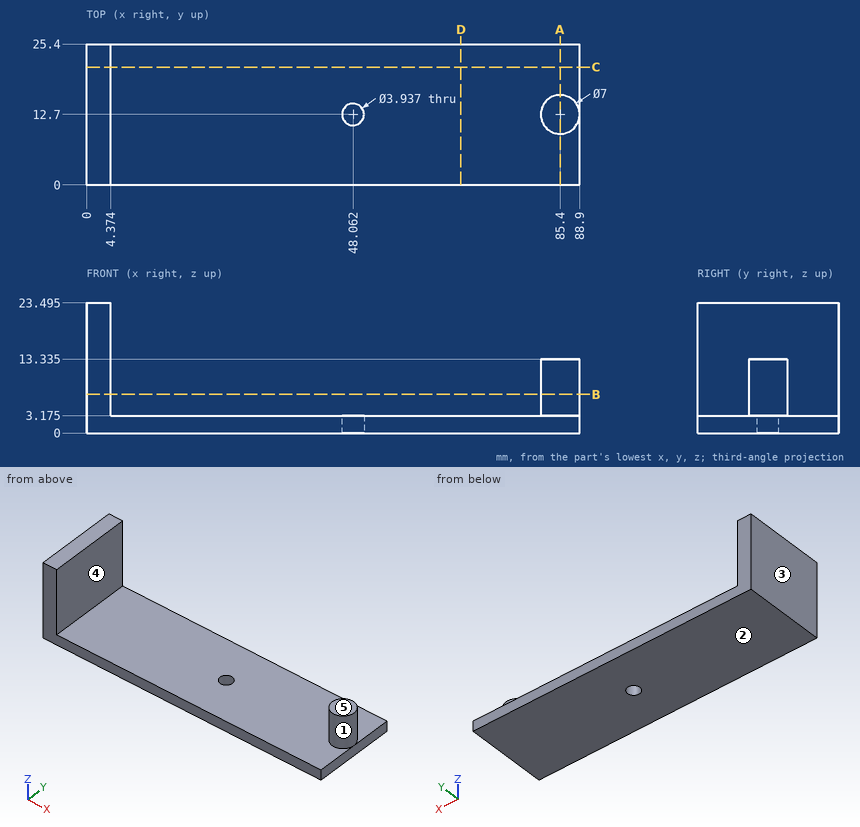
Answer from the drawing. Dimensions are ordinates in mm from the lowest x, y and z of the part. A direction names the side the tool comes from. Round coordinates to 2 decimals unless told otherwise and drop trailing zeros. Order: outer loops, then holes, each group sorted by start corner. A loop starts at its lowest first (then second) coordinate and runs counter-clockwise, first axis right, second up.
1) For the marked faces 4 and 5, determine the directions among +Z, -Z, +X, -X, +Y, -Y from which every point of the face is accessible in a straight line to the end or side of a thin tool.
2) The part is cut by section A-A on x = 85.4. Write down the section's boundary in (y, z) (3 decimals).
3) The part is cut by section C-C on y = 21.25. Write down the section's boundary in (x, z) (3 decimals).
4) The mould has two halves that part along X. Classify the marked faces 1, 2 and 3: released by +X, released by -X, zero draft, split by the parting line, or undercut.
5) Flat-ended cylindrical pins translate along their axes: pin 1 (7.5 mm diameter, centred on x = 86, y = 11.5, fed in from +Z) (3 decimals); pin 2 (2 mm diameter, centred on y = 20, z = 7.5, fed in from +X); pin 3 (7.5 mm diameter, centred on x = 48, y = 13.5, fed in from +Z) (3 decimals). Find the tip coordinate at first contact, or state that the pin passes through.
6) The part is cut by section B-B on z = 7. Write down the section's boundary in (x, y), plus the area to 3 significant figures.
7) The part is cut by section D-D on x = 67.5. Write down the section's boundary in (y, z) (3 decimals).
8) Straight lines are drawn through the part: L1, parallel to Z at x = 8.5, y = 14.5 (3 decimals); L2, parallel to X at y = 4.5, z = 7; L3, parallel to X at y = 13.5, z = 5.25. For each, find the intervals that lie inside material, in ascending order.
Resolved:
1. face 4: +Z, +Y, -Y
1. face 5: +Z, +X, +Y, -Y
2. outline: (0, 0) - (25.4, 0) - (25.4, 3.175) - (16.2, 3.175) - (16.2, 13.335) - (9.2, 13.335) - (9.2, 3.175) - (0, 3.175) - close
3. outline: (0, 0) - (88.9, 0) - (88.9, 3.175) - (4.374, 3.175) - (4.374, 23.495) - (0, 23.495) - close
4. face 1: undercut
4. face 2: zero draft
4. face 3: released by -X
5. pin 1: stops at z = 13.335
5. pin 2: stops at x = 4.37
5. pin 3: stops at z = 3.175
6. outline: (0, 0) - (4.37, 0) - (4.37, 25.4) - (0, 25.4) - close; circle Ø7 at (85.4, 12.7)
6. area: 150 mm2
7. outline: (0, 0) - (25.4, 0) - (25.4, 3.175) - (0, 3.175) - close
8. L1: z = 0 to 3.175
8. L2: x = 0 to 4.37
8. L3: x = 0 to 4.37, 81.99 to 88.81
